Input: dimensioned drawing with shaded views. Units: mm. Origin: part minimum x, y, z. A direction names the side the tool comes from. Coordinates: 2 decimals unless noted, no trailing zeros. Order: outer loops, then holes, each group sorted by start corner. A loop starts at its lowest first (then second) coordinate and runs counter-clockwise, first axis right, second up.
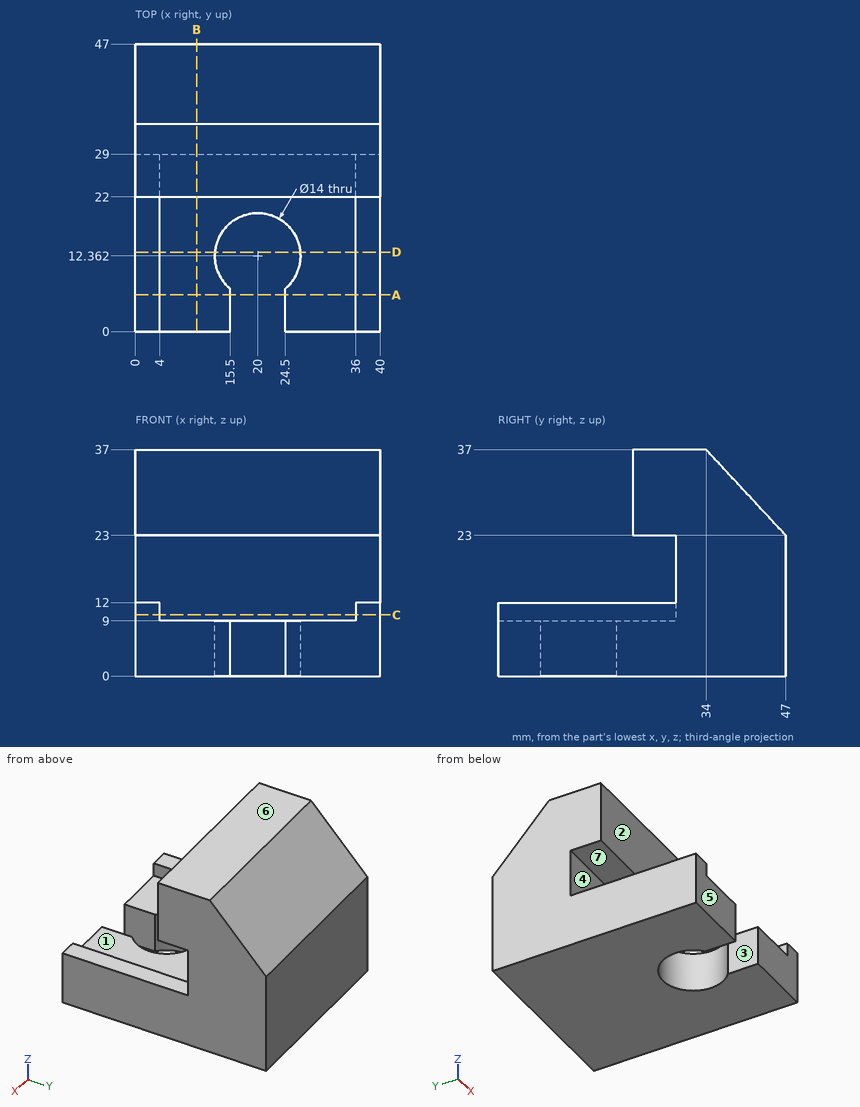
1. Draft query along Z for the marked faces 4, 5, 6 and 7. Return one class per face: released by +Z, released by -Z, zero draft, split by the parting line, or undercut.
Findings:
face 4: undercut
face 5: zero draft
face 6: released by +Z
face 7: undercut
2. Pin query (flat end, axial travel): P1, Ø8.5, axis at x = 24, y = 21, coming from the +Z side; P2, Ø5, axis at x = 34.5, z = 17.5, coming from the -Y side; P3, Ø10, axis at x = 28, z = 23.5, coming from the -Y side; P4, Ø2, axis at x = 37, y = 11.5, coming from the +Z side. Return the tip coordinate at first contact, or that it passes through.
Findings:
P1: stops at z = 37
P2: stops at y = 29
P3: stops at y = 22
P4: stops at z = 12
3. Ray query, line 1 (Z direction, x = 25, y = 26); line 2 (Z direction, x = 16, y = 18.5); line 3 (Y direction, x = 20, z = 5). Return the intervals inside material, ascending.
Findings:
line 1: z = 0 to 9, 23 to 37
line 2: z = 0 to 9
line 3: y = 19.36 to 47
4. Section query D-D on y = 13. Return loops of the section in (x, z).
Findings:
outline: (0, 0) - (13.03, 0) - (13.03, 9) - (4, 9) - (4, 12) - (0, 12) - close; (26.97, 0) - (40, 0) - (40, 12) - (36, 12) - (36, 9) - (26.97, 9) - close
5. Access query for the marked faces 1, 2 and 3. Directions: +Z, -Z, +X, -X, +Y, -Y. A direction counts if a zero-diameter tool reaches every point of the face in a straight line with its end or side. Return the directions, or none.
Findings:
face 1: -Y
face 2: +Z, +X, -X, -Y
face 3: +Z, -Z, -Y
6. Section query C-C on z = 10. Return loops of the section in (x, y).
Findings:
outline: (0, 0) - (4, 0) - (4, 29) - (36, 29) - (36, 0) - (40, 0) - (40, 47) - (0, 47) - close
7. Section query A-A on y = 6. Return loops of the section in (x, z).
Findings:
outline: (0, 0) - (15.5, 0) - (15.5, 9) - (4, 9) - (4, 12) - (0, 12) - close; (24.5, 0) - (40, 0) - (40, 12) - (36, 12) - (36, 9) - (24.5, 9) - close
8. Section query B-B on x = 10. Return loops of the section in (y, z), plus the area to 3 significant figures.
Findings:
outline: (0, 0) - (47, 0) - (47, 23) - (34, 37) - (22, 37) - (22, 23) - (29, 23) - (29, 9) - (0, 9) - close
area: 934 mm2
